```python
from build123d import *

# Parameters (mm, degrees)
SKETCH1_R           = 87.419609077
BOSS_EXTRUDE1_DEPTH = 61
FILLET1_R           = 30
SKETCH2_W           = 80
SKETCH2_H           = 49.2
CUT_EXTRUDE1_DEPTH  = 61


with BuildPart() as part:
    # Sketch1 → Boss-Extrude1 (new body)
    with BuildSketch(Plane.XY):
        with Locations(Location((0, 0, 0), (0, 0, 180))):
            Circle(SKETCH1_R)
    extrude(amount=BOSS_EXTRUDE1_DEPTH)

    # Fillet1
    fillet1_edges = [part.edges().sort_by_distance(p)[0] for p in [
        (87.419609077, 0, 61),
    ]]
    fillet(fillet1_edges, radius=FILLET1_R)

    # Sketch2 → Cut-Extrude1 (cut)
    with BuildSketch(Plane.XY.offset(61)):
        Rectangle(SKETCH2_W, SKETCH2_H)
    extrude(amount=-CUT_EXTRUDE1_DEPTH, mode=Mode.SUBTRACT)


solid = part.part
```
For this review, take the finished solid that the model builds, in its own axes (mm). A direction names the side the tool comes from. Coordinates: 2 decimals unless noted, no trailing zeros. Write each loop counter-clockwise with the first axis right and the second up, starting at its lowest first coordinate (ties: lowest second). Pieces come first, ordered by that corner, then holes. Notation, with made-up numbers: (13, 79) - (52, 79) arc R28 cw to (52, 104) - close; hole circle Ø10 at (-2, -12). An arc over 180 degrees is marked (long way). Put each result on its own line as item: value.
1. Machinability: for faces 4 (the flat face through (-1, -24.6, 31)), 5 (the flat face through (1, 25, 61)), which of the approach directions +Z, -Z, +X, -X, +Y, -Y give a long, thin tool a straight path to every point of the face, cutting with its end or side? Answer none if there is none.
Values found:
face 4: +Z, -Z
face 5: +Z, +X, -X, +Y, -Y
2. Mouldability with a two-part tool opening along X and no side actions: class faces 1 (the flat face through (40, 0, 31)), 2 (the flat face through (1, 38, 0)), 3 (the cylindrical face through (69.373, 53.193, 15.283)) as released by +X, released by -X, zero draft, split by the parting line, or undercut.
Values found:
face 1: undercut
face 2: zero draft
face 3: split by the parting line
3. Add section A-A, the plane x = 0. Give the boundary of the cut face in (y, z).
Values found:
outline: (-87.42, 0) - (-24.6, 0) - (-24.6, 61) - (-57.42, 61) arc R30 ccw to (-87.42, 31) - close; (24.6, 0) - (87.42, 0) - (87.42, 31) arc R30 ccw to (57.42, 61) - (24.6, 61) - close
4. Add section D-D, the plane z = 51.5. Give the boundary of the cut face in (x, y).
Values found:
outline: circle Ø158.65 at (0, 0); hole (-40, -24.6) - (40, -24.6) - (40, 24.6) - (-40, 24.6) - close
5. Add section B-B, the plane y = 0. Give the boundary of the cut face in (x, z).
Values found:
outline: (-87.42, 0) - (-40, 0) - (-40, 61) - (-57.42, 61) arc R30 ccw to (-87.42, 31) - close; (40, 0) - (87.42, 0) - (87.42, 31) arc R30 ccw to (57.42, 61) - (40, 61) - close
6. Add section C-C, the plane z = 4.5. Give the boundary of the cut face in (x, y).
Values found:
outline: circle Ø174.84 at (0, 0); hole (-40, -24.6) - (40, -24.6) - (40, 24.6) - (-40, 24.6) - close
7. Wall thickness on probe 1 along Y at (x, z) = (16.5, 52); probe 2 along X at (y, z) = (-22, 14); probe 3 along Y at (x, z) = (-37.5, 51): over which ranges is each line inside the solid? List them lowest first.
Values found:
probe 1: -77.1 to -24.6, 24.6 to 77.1
probe 2: -84.61 to -40, 40 to 84.61
probe 3: -70.42 to -24.6, 24.6 to 70.42
8. For pin 1 (12 mm diameter, centred on x = 24, z = 13.5, fed in from +Y); pin 2 (1.5 mm diameter, centred on y = 24, z = 20, fed in from +X); pin 3 (10 mm diameter, centred on x = -57.5, z = 37, fed in from +Y), all flat-tipped, find the tip position at first contact; note any pin that passes through.
Values found:
pin 1: y = 85.55
pin 2: x = 84.27
pin 3: y = 69.31
